Source: CAD feature listing. Evaluate the final solid. Frame: model axes, mm. A direction names the side the tool comes from. Give positions to 0.01 mm unless a question says otherwise; leave off trailing zeros. Write each loop counter-clockwise with the first axis right and the second up, starting at its lowest first coordinate (ties: lowest second). Pieces come first, ordered by that corner, then holes. Notation, with made-up numbers: M 48,81 L 100,81 A20 ccw 100,93 Z; hole C 87,45 d2. An arc over 180 degrees is marked long. Answer as a JSON object with one key per item and string values. Group by question number.
```python
from build123d import *

# Parameters (mm, degrees)
F0_W     = 80
F0_H     = 80
F3_DEPTH = 25
F4_T     = -15
F1_W     = 2
F1_H     = 48
F2_W     = 2
F2_H     = 48
F6_DEPTH = 25
F7_D     = 2
F9_D     = 5


with BuildPart() as f3:
    # F0 (on Top) → F3 (new body)
    with BuildSketch(Plane.XY):
        Rectangle(F0_W, F0_H)
    extrude(amount=F3_DEPTH)

    # F4
    f4_openings = [f3.faces().sort_by_distance(p)[0] for p in [
        (0, 0, 25),
    ]]
    offset(amount=F4_T, openings=f4_openings)

    # F1 (on face) + F2 (on face) → F6 (join)
    with BuildSketch(Plane.XY):
        with Locations((-21.533683, 1.29566)):
            Rectangle(F1_W, F1_H)
    with BuildSketch(Plane.XY):
        with Locations((-17.357037, -1.363026)):
            Rectangle(F2_W, F2_H)
        with Locations((-13.159431, 1.430389)):
            Rectangle(F2_W, F2_H)
        with Locations((-8.982785, -1.363026)):
            Rectangle(F2_W, F2_H)
        with Locations((-4.940869, 1.29566)):
            Rectangle(F2_W, F2_H)
        with Locations((-1, -1.228295)):
            Rectangle(F2_W, F2_H)
        with Locations((3.412425, 1.160929)):
            Rectangle(F2_W, F2_H)
        with Locations((8.127995, -1.363026)):
            Rectangle(F2_W, F2_H)
        with Locations((12.304641, 1.331586)):
            Rectangle(F2_W, F2_H)
        with Locations((16.481286, -1.228295)):
            Rectangle(F2_W, F2_H)
        with Locations((21.466319, 1.331586)):
            Rectangle(F2_W, F2_H)
    extrude(amount=F6_DEPTH)

    # F7 (through all)
    with Locations(Plane.XY.offset(15)):
        with Locations((-23.611529, 23.544163), (23.678893, 23.409432)):
            Hole(F7_D / 2)

    # F9 (through all)
    with Locations(Plane.XY.offset(25)):
        with Locations((-34.25524, 34.592066), (34.8069, 35.473198), (34.113035, -34.558825), (-34.355238, -34.1)):
            Hole(F9_D / 2)


solid = f3.part
```
(1) Contact query for a flat-ended pin moving along its axis: pin 1 Ø1.8 at (x, y) = (23.68, 23.41) entering from +Z. Output: stop coordinate, or through.
(2) Section A-A, the plane x = 19. Return loops of the section in (y, z), plus the area to 3 significant figures.
(3) Ray query, L1, parallel to X at y = -34, z = 20.5; L2, parallel to Y at x = 34.5, z = 9.75; L3, parallel to Y at x = -24, z = 17. Return the intervals inside material, ascending. Write a range as [from, to].
(4) Access query for faces 1 (the cylindrical face through (-24.073, 22.657, 7.395)), 2 (the flat face through (-1, 22.772, 20)). Directions: +Z, -Z, +X, -X, +Y, -Y. A direction counts if a zero-diameter tool reaches every point of the face in a straight line with its end or side. Return the directions, or none.
(5) Section B-B, the plane z = 23.25. State how many separate pieces and enclosed holes the cut face has, plus the area to 3 significant figures.
(6) Pull-direction query (Y, two-part tool) for faces 3 (the flat face through (-1, 1, 0)), 4 (the flat face through (-22, -25, 20)); classes: pulls with the +Y half, pulls with the -Y half, needs draft (parallel to the pull), parting line crosses it, or undercut.
Reported:
{
 "1": {"pin 1": "passes through"},
 "2": {"outline": "M -40,0 L 40,0 L 40,25 L 25,25 L 25,15 L -25,15 L -25,25 L -40,25 Z", "area": "1,500 mm2"},
 "3": {"L1": "x = [-40, -36.85], [-31.86, 31.68], [36.55, 40]", "L2": "y = [-40, -37.03], [-32.09, 32.99], [37.95, 40]", "L3": "y = [-40, -25], [25, 40]"},
 "4": {"face 1": "+Z, -Z", "face 2": "+Z"},
 "5": {"separate pieces": "1", "enclosed holes": "5", "area": "4,870 mm2"},
 "6": {"face 3": "needs draft", "face 4": "undercut"}
}
